from build123d import *

# Parameters (mm, degrees)
SKETCH2_W           = 180
SKETCH2_H           = 190
BOSS_EXTRUDE3_DEPTH = 5
SKETCH4_W           = 5
SKETCH4_H           = 190
BOSS_EXTRUDE4_DEPTH = 50
SKETCH6_W           = 250
SKETCH6_H           = 3.1090482
BOSS_EXTRUDE6_DEPTH = 80
SKETCH7_W           = 35
SKETCH7_H           = 78.948410215
SKETCH7_H_2         = 80
BOSS_EXTRUDE7_DEPTH = 50
SKETCH8_W           = 80
SKETCH8_H           = 3.1090482
CUT_EXTRUDE1_DEPTH  = 123
SKETCH9_W           = 80
SKETCH9_H           = 50
CUT_EXTRUDE2_DEPTH  = 123
BOSS_EXTRUDE8_DEPTH = 75


with BuildPart() as part:
    # Sketch2 → Boss-Extrude3 (new body)
    with BuildSketch(Plane(origin=(0, 0, 0), x_dir=(1, 0, 0), z_dir=(0, 1, 0))):
        Rectangle(SKETCH2_W, SKETCH2_H)
    extrude(amount=BOSS_EXTRUDE3_DEPTH)

    # Sketch4 → Boss-Extrude4 (add)
    with BuildSketch(Plane(origin=(0, 5, 0), x_dir=(1, 0, 0), z_dir=(0, 1, 0))):
        with Locations((-87.5, 0)):
            Rectangle(SKETCH4_W, SKETCH4_H)
        with Locations((87.5, 0)):
            Rectangle(SKETCH4_W, SKETCH4_H)
    extrude(amount=BOSS_EXTRUDE4_DEPTH)

    # Sketch6 → Boss-Extrude6 (add)
    with BuildSketch(Plane(origin=(0, 0, 0), x_dir=(1, 0, 0), z_dir=(0, 1, 0))):
        with Locations((0, 96.5545241)):
            Rectangle(SKETCH6_W, SKETCH6_H)
    extrude(amount=BOSS_EXTRUDE6_DEPTH)

    # Sketch7 → Boss-Extrude7 (add)
    with BuildSketch(Plane(origin=(0, 0, -98.1090482), x_dir=(-1, 0, 0), z_dir=(0, 0, -1))):
        with Locations((-57.5, 39.474205108)):
            Rectangle(SKETCH7_W, SKETCH7_H)
        with Locations((57.5, 40)):
            Rectangle(SKETCH7_W, SKETCH7_H_2)
    extrude(amount=BOSS_EXTRUDE7_DEPTH)

    # Sketch8 → Cut-Extrude1 (cut)
    with BuildSketch(Plane(origin=(0, 80, 0), x_dir=(1, 0, 0), z_dir=(0, 1, 0))):
        with Locations((0, 96.5545241)):
            Rectangle(SKETCH8_W, SKETCH8_H)
    extrude(amount=-CUT_EXTRUDE1_DEPTH, mode=Mode.SUBTRACT)

    # Sketch9 → Cut-Extrude2 (cut)
    with BuildSketch(Plane(origin=(0, 5, 0), x_dir=(1, 0, 0), z_dir=(0, 1, 0))):
        with Locations((0, 70)):
            Rectangle(SKETCH9_W, SKETCH9_H)
    extrude(amount=-CUT_EXTRUDE2_DEPTH, mode=Mode.SUBTRACT)

    # Sketch10 → Boss-Extrude8 (add)
    with BuildSketch(Plane(origin=(0, 5, 0), x_dir=(1, 0, 0), z_dir=(0, 1, 0))):
        Polygon((-40, 95), (-40, 45), (40, 45), (40, 95), (45, 95), (45, 40), (-45, 40), (-45, 95), align=None)
    extrude(amount=BOSS_EXTRUDE8_DEPTH)


solid = part.part
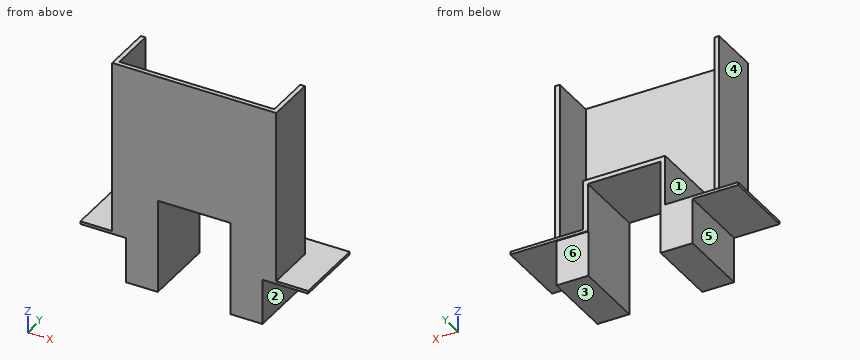
Model file for the job. Use its own axes, mm. Face numbers are marked on the shaded views. A direction names the side the tool comes from. Coordinates: 2 decimals unless noted, no trailing zeros. Write each loop counter-clockwise with the first axis right and the second up, starting at its lowest first coordinate (ties: lowest second). Pieces come first, ordered by that corner, then holes. Notation, with made-up numbers: (66, 20) -> (74, 20) arc R18 cw to (74, 49) -> close; hole circle Ø7 at (18.25, 0). An arc over 180 degrees is marked (long way). One line per item, written item: value. Start each with the question number.
1) Slice it at A-A on z = -101.5. Write the cut outline in (x, y), then the cut area to 3 significant figures.
2) Probe probe 1 along X at (y, z) = (33, -91.5); probe 2 along X at (y, z) = (8, -114); probe 3 along X at (y, z) = (38.5, -27). List the from-to ranges inside material, lowest first.
3) Slice it at C-C on y = 44. Write the cut outline in (x, z), then the cut area to 3 significant figures.
4) Which spindle directions (+Z, -Z, +X, -X, +Y, -Y) get a long thin tool onto all of the face, cutting with end or side? Do the marked faces 4, 5 and 6. Say none if no direction does.
5) Slice it at D-D on z = -37. Write the cut outline in (x, y), then the cut area to 3 significant figures.
6) Slice it at B-B on x = 55.5. Write the cut outline in (y, z).
7) Pull direction X, two halves, no side cores. Call the marked faces 1, 2 and 3: +X half, -X half, draft (parallel to the pull), parting line (faces both ways), or undercut.
8) Flat gauge pins, fed straight in: pin 1 Ø1 at (x, y) = (22, 33.5) entering from -Z; pin 2 Ø15 at (y, z) = (49.5, -112.5) entering from -X; pin 3 Ø10 at (x, z) = (-85.5, 60) entering from +Y. Where does each tip first touch, or does it go through?
Answers follow:
1. outline: (-75, 0) -> (-40, 0) -> (-40, 80) -> (-75, 80) -> close; (40, 0) -> (75, 0) -> (75, 78.95) -> (40, 78.95) -> close
1. area: 5,560 mm2
2. probe 1: -90 to -85, -45 to -40, 40 to 45, 85 to 90
2. probe 2: -75 to -40, 40 to 75
2. probe 3: -90 to -85, 85 to 90
3. outline: (-125, -98.11) -> (-75, -98.11) -> (-75, -148.11) -> (-40, -148.11) -> (-40, -45) -> (40, -45) -> (40, -148.11) -> (75, -148.11) -> (75, -98.11) -> (125, -98.11) -> (125, -95) -> (90, -95) -> (90, 95) -> (85, 95) -> (85, -95) -> (45, -95) -> (45, -40) -> (-45, -40) -> (-45, -95) -> (-85, -95) -> (-85, 95) -> (-90, 95) -> (-90, -95) -> (-125, -95) -> close
3. area: 6,880 mm2
4. face 4: +Z, -X, +Y, -Y
4. face 5: -Z, -X, +Y, -Y
4. face 6: -Z, +X, +Y
5. outline: (-90, 0) -> (90, 0) -> (90, 55) -> (85, 55) -> (85, 5) -> (-85, 5) -> (-85, 55) -> (-90, 55) -> close
5. area: 1,400 mm2
6. outline: (0, -148.11) -> (78.95, -148.11) -> (78.95, -98.11) -> (80, -98.11) -> (80, -95) -> (5, -95) -> (5, 95) -> (0, 95) -> close
7. face 1: undercut
7. face 2: +X half
7. face 3: draft
8. pin 1: z = -45
8. pin 2: x = -75
8. pin 3: y = 55
